Here's how the part is built. I have some questions about the finished solid (model axes, mm). A direction names the side the tool comes from. Coordinates: 2 decimals unless noted, no trailing zeros. Write each loop counter-clockwise with the first axis right and the second up, starting at its lowest first coordinate (ties: lowest second). Pieces come first, ordered by that corner, then holes. Notation, with made-up numbers: (81.5, -8) -> (85.5, -8) arc R22 cw to (85.5, 0) -> close; hole circle Ø10 at (18.25, 70.5). An arc over 180 degrees is marked (long way). Put each result on its own line as item: value.
```python
from build123d import *

# Parameters (mm, degrees)
F0_W     = 15
F0_H     = 7.8
F0_R     = 2.1
F0_W_2   = 7.8
F0_H_2   = 14.85
F0_R_2   = 2.8
F1_DEPTH = 10
F2_START = 9
F2_DEPTH = 2
F3_START = 3.8
F3_DEPTH = 4.2
F4_SIZE  = 2


with BuildPart() as f1:
    # F0 (on Top) → F1 (new body)
    with BuildSketch(Plane.XY):
        Polygon((7.4437668294, -7.943718292), (7.4437668294, 6.906281708), (15.2437668294, 6.906281708), (15.2437668294, 12.056281708), (-18.8392331706, 12.056281708), (-18.8392331706, 9.493718292), (-3.8392331706, 9.493718292), (-3.8392331706, 1.693718292), (-18.8392331706, 1.693718292), (-18.8392331706, -7.943718292), align=None)
        Polygon((15.2437668294, -7.943718292), (7.4437668294, -7.943718292), (7.4437668294, -10.4582807188), (11.3013526795, -8.186424295), (15.2437668294, -10.4173709361), align=None)
        Polygon((7.115132639, -15.5840970217), (7.0875579305, -12.393718292), (3.9437668294, -12.393718292), (7.115132639, -17.5585140392), align=None)
        Polygon((7.4437668294, -18.093718292), (7.4437668294, -15.7700656479), (7.115132639, -15.5840970217), (7.115132639, -17.5585140392), align=None)
        Polygon((18.7437668294, -12.393718292), (15.5878754119, -12.393718292), (15.6148151695, -15.5106335593), (15.6148151695, -17.4894395666), align=None)
        Polygon((15.6148151695, -15.5106335593), (15.2437668294, -15.7291558652), (15.2437668294, -18.093718292), (15.6148151695, -17.4894395666), align=None)
        with Locations((-11.3392331706, 5.593718292)):
            Rectangle(F0_W, F0_H)
        with Locations((-14.3314907327, 5.593718292)):
            Circle(F0_R, mode=Mode.SUBTRACT)
        with Locations((11.3437668294, -0.518718292)):
            Rectangle(F0_W_2, F0_H_2)
        with Locations((11.3437668294, 2.4854193907)):
            Circle(F0_R, mode=Mode.SUBTRACT)
        Polygon((11.3861809792, -18.001012289), (7.4437668294, -15.7700656479), (7.4437668294, -18.093718292), (15.2437668294, -18.093718292), (15.2437668294, -15.7291558652), align=None)
        Polygon((7.4437668294, -15.7700656479), (7.4437668294, -12.393718292), (7.0875579305, -12.393718292), (7.115132639, -15.5840970217), align=None)
        Polygon((15.5878754119, -12.393718292), (15.2437668294, -12.393718292), (15.2437668294, -15.7291558652), (15.6148151695, -15.5106335593), align=None)
        Polygon((11.3013526795, -8.186424295), (7.4437668294, -10.4582807188), (7.4437668294, -12.393718292), (7.4437668294, -15.7700656479), (11.3861809792, -18.001012289), (15.2437668294, -15.7291558652), (15.2437668294, -12.393718292), (15.2437668294, -10.4173709361), align=None)
        with Locations((11.3437668294, -13.093718292)):
            Circle(F0_R_2, mode=Mode.SUBTRACT)
    extrude(amount=F1_DEPTH)

    # F0 (on Top) → F2 (join)
    with BuildSketch(Plane.XY.offset(F2_START)):
        with Locations((-11.3392331706, 5.593718292)):
            Rectangle(F0_W, F0_H)
        with Locations((-14.3314907327, 5.593718292)):
            Circle(F0_R, mode=Mode.SUBTRACT)
        with Locations((11.3437668294, -0.518718292)):
            Rectangle(F0_W_2, F0_H_2)
        with Locations((11.3437668294, 2.4854193907)):
            Circle(F0_R, mode=Mode.SUBTRACT)
        Polygon((7.4437668294, -15.7700656479), (7.4437668294, -12.393718292), (7.0875579305, -12.393718292), (7.115132639, -15.5840970217), align=None)
        Polygon((7.4437668294, -18.093718292), (7.4437668294, -15.7700656479), (7.115132639, -15.5840970217), (7.115132639, -17.5585140392), align=None)
        Polygon((11.3861809792, -18.001012289), (7.4437668294, -15.7700656479), (7.4437668294, -18.093718292), (15.2437668294, -18.093718292), (15.2437668294, -15.7291558652), align=None)
        Polygon((18.7437668294, -12.393718292), (15.5878754119, -12.393718292), (15.6148151695, -15.5106335593), (15.6148151695, -17.4894395666), align=None)
        Polygon((15.6148151695, -15.5106335593), (15.2437668294, -15.7291558652), (15.2437668294, -18.093718292), (15.6148151695, -17.4894395666), align=None)
        Polygon((7.115132639, -15.5840970217), (7.0875579305, -12.393718292), (3.9437668294, -12.393718292), (7.115132639, -17.5585140392), align=None)
        Polygon((11.3013526795, -8.186424295), (7.4437668294, -10.4582807188), (7.4437668294, -12.393718292), (7.4437668294, -15.7700656479), (11.3861809792, -18.001012289), (15.2437668294, -15.7291558652), (15.2437668294, -12.393718292), (15.2437668294, -10.4173709361), align=None)
        with Locations((11.3437668294, -13.093718292)):
            Circle(F0_R_2, mode=Mode.SUBTRACT)
        Polygon((15.2437668294, -7.943718292), (7.4437668294, -7.943718292), (7.4437668294, -10.4582807188), (11.3013526795, -8.186424295), (15.2437668294, -10.4173709361), align=None)
        Polygon((15.5878754119, -12.393718292), (15.2437668294, -12.393718292), (15.2437668294, -15.7291558652), (15.6148151695, -15.5106335593), align=None)
    extrude(amount=F2_DEPTH)

    # F0 (on Top) → F3 (cut)
    with BuildSketch(Plane.XY.offset(F3_START)):
        Polygon((15.5724010197, -10.6033395623), (15.2437668294, -10.4173709361), (15.2437668294, -12.393718292), (15.5878754119, -12.393718292), align=None)
        Polygon((11.3013526795, -8.186424295), (7.4437668294, -10.4582807188), (7.4437668294, -12.393718292), (7.4437668294, -15.7700656479), (11.3861809792, -18.001012289), (15.2437668294, -15.7291558652), (15.2437668294, -12.393718292), (15.2437668294, -10.4173709361), align=None)
        with Locations((11.3437668294, -13.093718292)):
            Circle(F0_R_2, mode=Mode.SUBTRACT)
        Polygon((15.5878754119, -12.393718292), (15.2437668294, -12.393718292), (15.2437668294, -15.7291558652), (15.6148151695, -15.5106335593), align=None)
        Polygon((7.4437668294, -15.7700656479), (7.4437668294, -12.393718292), (7.0875579305, -12.393718292), (7.115132639, -15.5840970217), align=None)
        Polygon((7.4437668294, -12.393718292), (7.4437668294, -10.4582807188), (7.0727184892, -10.6768030247), (7.0875579305, -12.393718292), align=None)
        Polygon((11.3861809792, -18.001012289), (7.4437668294, -15.7700656479), (7.4437668294, -18.093718292), (15.2437668294, -18.093718292), (15.2437668294, -15.7291558652), align=None)
        Polygon((15.6148151695, -15.5106335593), (15.2437668294, -15.7291558652), (15.2437668294, -18.093718292), (15.6148151695, -17.4894395666), align=None)
        Polygon((7.4437668294, -18.093718292), (7.4437668294, -15.7700656479), (7.115132639, -15.5840970217), (7.115132639, -17.5585140392), align=None)
    extrude(amount=F3_DEPTH, mode=Mode.SUBTRACT)

    # F4
    f4_edges = [f1.edges().sort_by_distance(p)[0] for p in [
        (15.243767, 12.056282, 5),
        (-18.839233, -7.943718, 5),
        (-18.839233, 12.056282, 5),
    ]]
    chamfer(f4_edges, length=F4_SIZE)


solid = f1.part
```
Item 1: For P1, Ø5, axis at x = -0.5, z = 5, coming from the -Y side; P2, Ø3, axis at x = -5.5, y = -10, coming from the +Z side; P3, Ø0.6, axis at y = -17, z = 5.5, coming from the +X side; P4, Ø1.1, axis at y = 4.5, z = 10.5, coming from the +X side, each with a flat end and sliding along its axis, tell me the tip position at first contact or that it passes through.
Output:
P1: stops at y = -7.94
P2: passes through
P3: stops at x = 16.1
P4: stops at x = 15.24
Item 2: If we mould it in two halves opening along Z, with no side actions, what happens to faces 5 (the flat face through (6, -12.394, 5)), 6 (the flat face through (9, -15, 3.8)), 7 (the flat face through (13.3, -9.318, 5.871)), 8 (the flat face through (-11, 6, 11))? For each: released by +Z, released by -Z, zero draft, split by the parting line, or undercut.
Output:
face 5: zero draft
face 6: undercut
face 7: undercut
face 8: released by +Z
Item 3: Imagine slicing it at A-A on z = 5.75. Write out the boundary of the cut face in (x, y).
Output:
outline: (-18.84, -5.94) -> (-16.84, -7.94) -> (7.44, -7.94) -> (7.44, -10.46) -> (11.3, -8.19) -> (15.24, -10.42) -> (15.24, 10.06) -> (13.24, 12.06) -> (-16.84, 12.06) -> (-18.84, 10.06) -> close; (3.94, -12.39) -> (7.12, -17.56) -> (7.12, -15.58) -> (7.09, -12.39) -> close; (15.59, -12.39) -> (15.61, -15.51) -> (15.61, -17.49) -> (18.74, -12.39) -> close; hole circle Ø4.2 at (-14.33, 5.59); hole circle Ø4.2 at (11.34, 2.49)
Item 4: Please list where these lines run through material, in increasing order: line 1 along Z through (x, y) = (11, -17); line 2 along Z through (x, y) = (9, 9); line 3 along Y through (x, z) = (-2, 7). Write a range as from..to.
Output:
line 1: z = 0..3.8, 8..11
line 2: z = 0..10
line 3: y = -7.94..12.06
Item 5: Imagine slicing it at B-B on y = -11.5. Write out the boundary of the cut face in (x, z), then the cut area to 3 significant figures.
Output:
outline: (7.44, 0) -> (9.04, 0) -> (9.04, 3.8) -> (7.44, 3.8) -> close; (7.44, 8) -> (9.04, 8) -> (9.04, 11) -> (7.44, 11) -> close; (13.65, 0) -> (15.24, 0) -> (15.24, 3.8) -> (13.65, 3.8) -> close; (13.65, 8) -> (15.24, 8) -> (15.24, 11) -> (13.65, 11) -> close
area: 21.7 mm²
Item 6: Imagine slicing it at D-D on z = 1. Write out the boundary of the cut face in (x, y).
Output:
outline: (-18.84, -5.94) -> (-16.84, -7.94) -> (7.44, -7.94) -> (7.44, -12.39) -> (3.94, -12.39) -> (7.44, -18.09) -> (15.24, -18.09) -> (18.74, -12.39) -> (15.24, -12.39) -> (15.24, 10.06) -> (13.24, 12.06) -> (-16.84, 12.06) -> (-18.84, 10.06) -> close; hole circle Ø4.2 at (-14.33, 5.59); hole circle Ø5.6 at (11.34, -13.09); hole circle Ø4.2 at (11.34, 2.49)
Item 7: Imagine slicing it at C-C on x = -8.5. Write out the boundary of the cut face in (y, z), then the cut area to 3 significant figures.
Output:
outline: (-7.94, 0) -> (12.06, 0) -> (12.06, 10) -> (9.49, 10) -> (9.49, 11) -> (1.69, 11) -> (1.69, 10) -> (-7.94, 10) -> close
area: 208 mm²
Item 8: Which directions (+Z, -Z, +X, -X, +Y, -Y) give clear straight access to the entire face, cutting with the end or side of a thin tool? Please do faces 1 (the flat face through (-3.839, 5.5, 10.5)), 2 (the flat face through (17, -12.394, 5)), 3 (the flat face through (11.3, 6.906, 10.5)), 4 (the flat face through (-11.4, 9.494, 10.5)).
Output:
face 1: +Z, +Y, -Y
face 2: +Z, -Z, +X, +Y
face 3: +Z, +X, +Y
face 4: +Z, +X, -X, +Y
